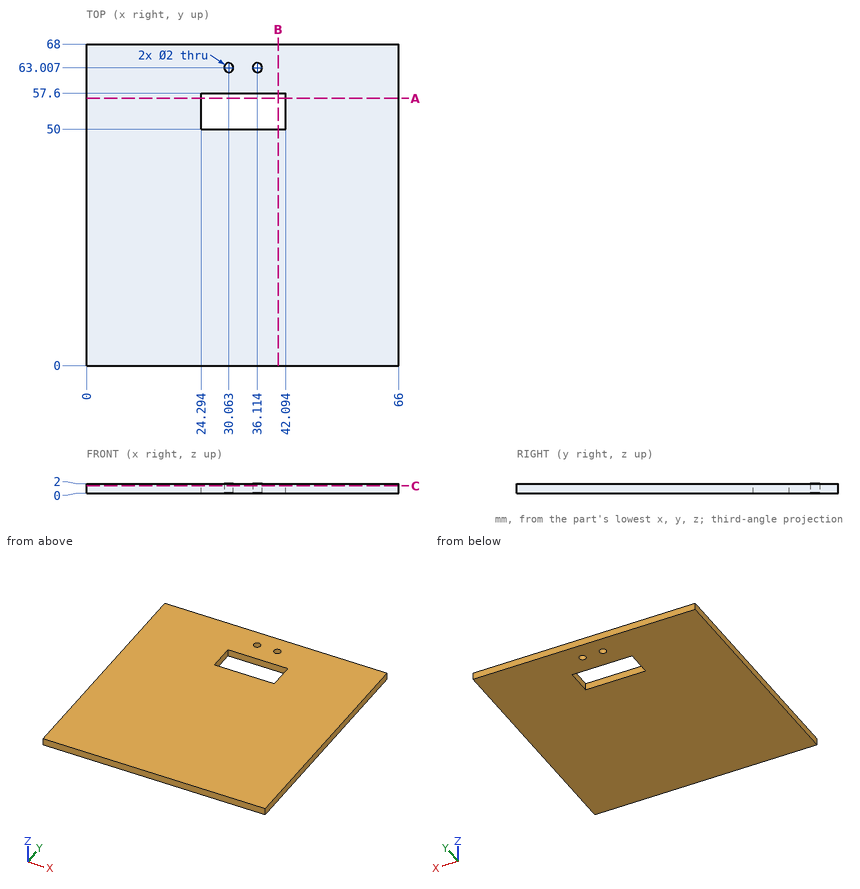
Drawing for the job (mm, zero at the part's lowest x, y, z). Give positions to 0.01 mm unless a question says otherwise; leave off trailing zeros. Order: outer loops, then holes, each group sorted by start corner. A loop starts at its lowest first (then second) coordinate and runs counter-clockwise, first axis right, second up. Notation, with made-up numbers: M 81.25,33 L 92.25,33 A14 ccw 92.25,39 Z; hole C 44.5,71.5 d5. An arc over 180 degrees is marked long. Write item = value, one per line. Start each with the question number.
(1) Slice it at A-A on y = 56.5. Write the cut outline in (x, z) (1 decimal).
(2) Pin check, flat tip, straight feed: pin 1 Ø1 at (x, z) = (35, 0.5) entering from -Y. Stop position of the tip, or through.
(3) Slice it at C-C on z = 1.55. Write the cut outline in (x, y) (1 decimal), plus the area to 3 significant figures.
(4) Probe L1, parallel to X at y = 53, z = 1.5 (1 decimal); L2, parallel to Y at x = 25, z = 0.85; L3, parallel to Y at x = 29.5, z = 0.2 (1 decimal). List the from-to ranges inside material, lowest first. Write a range as [from, to].
(5) Slice it at B-B on x = 40.5. Write the cut outline in (y, z).
Responses:
q1.outline = M 0,0 L 24.3,0 L 24.3,2 L 0,2 Z; M 42.1,0 L 66,0 L 66,2 L 42.1,2 Z
q2.pin_1 = 0
q3.outline = M 0,0 L 66,0 L 66,68 L 0,68 Z; hole M 24.3,50 L 42.1,50 L 42.1,57.6 L 24.3,57.6 Z; hole C 30.1,63 d2; hole C 36.1,63 d2
q3.area = 4,350 mm2
q4.L1 = [0, 24.3], [42.1, 66]
q4.L2 = [0, 50], [57.6, 68]
q4.L3 = [0, 50], [57.6, 62.2], [63.8, 68]
q5.outline = M 0,0 L 50,0 L 50,2 L 0,2 Z; M 57.6,0 L 68,0 L 68,2 L 57.6,2 Z
